The listing builds one solid part. Answer for the finished solid, in the listing's coordinates (mm). A direction names the side the tool comes from. Coordinates: 2 decimals unless noted, no trailing zeros. Order: outer loops, then holes, each group sorted by start corner. A loop starts at its lowest first (then second) coordinate and runs counter-clockwise, first axis right, second up. Notation, with made-up numbers: (56.5, 33.25) - (112.5, 33.25) arc R29 ccw to (112.5, 57.25) - close; hole circle Ø10 at (23.25, 70.5). An arc over 180 degrees is marked (long way). Use a Markdown table: item, result. Add a question column.
Item 1: The part is cut by section D-D, the plane z = -15. Give the vertices of the cut face in (x, y).
Item 2: The part is cut by section A-A, the plane x = 0. Give the vertices of the cut face in (y, z).
Item 3: The mould has two halves that part along X. Classify faces 1 (the flat face through (-1, 1, 51.235)), 2 (the flat face through (-17, 2, 18.867)), 3 (the cylindrical face through (31.29, 1.479, -44.397)), 4 (the flat face through (40, 2, 1)): released by +X, released by -X, zero draft, split by the parting line, or undercut.
Item 4: Flat-ended cylindrical pins translate along their axes: P1, Ø6, axis at x = 3, z = -2, coming from the -Y side; P2, Ø7, axis at x = 32.5, z = 42.5, coming from the +Y side; P3, Ø4, axis at x = -32.5, z = 42.5, coming from the -Y side. Find the tip coordinate at first contact, or state that the pin passes through.
Item 5: Find the intervals of material crossed by line 1 along X through (y, z) = (1.75, 42.5); line 2 along Z through (x, y) = (30, 1.75); line 3 along Y through (x, z) = (-5.5, 30.5), in increasing order.
Item 6: For faces 5 (the flat face through (0, 3, -39)), 6 (the flat face through (-1, 0, -12)), 7 (the flat face through (22.25, 2, -38)), determine the directions among +Z, -Z, +X, -X, +Y, -Y from which every point of the face is accessible in a straight line to the end or side of a thin tool.
Item 7: The part is cut by section B-B, the plane z = -39. Give the vertices of the cut face in (x, y).
Item 8: The part is cut by section C-C, the plane x = 16.5. Give the vertices of the cut face in (y, z), then the cut area to 3 significant figures.
from build123d import *

# Parameters (mm, degrees)
ESQUISSE1_R             = 65
DISQUE_DEPTH            = 3
ESQUISSE3_W             = 30.466369815
ESQUISSE3_H             = 200
COT_S_DEPTH             = 4
D_GAGEMENT_M3_52_D      = 3.9
D_GAGEMENT_M42_D        = 4.5
ESQUISSE15_W            = 89.863216067
ESQUISSE15_H            = 32.096215679
ENL_V_MAT_EXTRU_1_DEPTH = 34
D_GAGEMENT_M3_53_D      = 3.9
D_GAGEMENT_M3_53_DEPTH  = 3
D_GAGEMENT_M3_53_TIP    = 1.171678207
ESQUISSE22_W            = 113.248519978
ESQUISSE22_H            = 34.612898142
ESQUISSE22_W_2          = 51
ESQUISSE22_H_2          = 7
ESQUISSE22_W_3          = 65
ESQUISSE22_H_3          = 8
ENL_V_MAT_EXTRU_3_DEPTH = 10
ESQUISSE23_W            = 12
ESQUISSE23_H            = 14
ENL_V_MAT_EXTRU_4_DEPTH = 10
ESQUISSE24_W            = 18
ESQUISSE24_H            = 15
ENL_V_MAT_EXTRU_5_DEPTH = 10


with BuildPart() as part:
    # Esquisse1 → disque (new body)
    with BuildSketch(Plane(origin=(0, 0, 0), x_dir=(1, 0, 0), z_dir=(0, 1, 0))):
        Circle(ESQUISSE1_R)
    extrude(amount=DISQUE_DEPTH)

    # Esquisse3 → cotés (cut, through all)
    with BuildSketch(Plane(origin=(0, 3, 0), x_dir=(1, 0, 0), z_dir=(0, 1, 0))):
        with Locations((-55.233184908, 0)):
            Rectangle(ESQUISSE3_W, ESQUISSE3_H)
        with Locations((55.233184908, 0)):
            Rectangle(ESQUISSE3_W, ESQUISSE3_H)
    extrude(amount=-COT_S_DEPTH, mode=Mode.SUBTRACT)

    # Dégagement M3.52 (through all)
    with Locations(Plane(origin=(0, 3, 0), x_dir=(1, 0, 0), z_dir=(0, 1, 0))):
        with Locations((-30, -28.76524617)):
            d_gagement_m3_52 = Hole(D_GAGEMENT_M3_52_D / 2)

    # Symétrie1: Dégagement M3.52 across plane
    add(d_gagement_m3_52.mirror(Plane.ZY), mode=Mode.SUBTRACT)

    # Dégagement M42 (through all)
    with Locations(Plane(origin=(0, 3, 0), x_dir=(1, 0, 0), z_dir=(0, 1, 0))):
        with Locations((-32.5, 42.5), (32.5, 42.5), (32.5, -42.5), (-32.5, -42.5)):
            Hole(D_GAGEMENT_M42_D / 2)

    # Esquisse14 → Révolution1 (revolve)
    with BuildSketch(Plane.ZY):
        with BuildLine():
            Line((-35, 3), (-32, 3))
            Line((-32, 3), (-32, 26))
            ThreePointArc((-32, 26), (-34.050252532, 30.949747468), (-39, 33))
            Line((-39, 33), (-39, 30))
            ThreePointArc((-39, 30), (-36.171572875, 28.828427125), (-35, 26))
            Line((-35, 26), (-35, 3))
        make_face()
    revolve(axis=Axis((0, 3, -39), (0, 1, 0)))

    # Esquisse15 → Enlèv. mat.-Extru.1 (cut, through all)
    with BuildSketch(Plane.XZ):
        with Locations((-4.931608034, 67.282861669)):
            Rectangle(ESQUISSE15_W, ESQUISSE15_H)
    extrude(amount=-ENL_V_MAT_EXTRU_1_DEPTH, mode=Mode.SUBTRACT)

    # Dégagement M3.53
    with Locations(Plane(origin=(0, 0, 0), x_dir=(-1, 0, 0), z_dir=(0, -1, 0))):
        with Locations((-11.313708499, -8.367376915), (11.313708499, -36.367376915)):
            Hole(D_GAGEMENT_M3_53_D / 2, depth=D_GAGEMENT_M3_53_DEPTH)
            with Locations((0, 0, -(D_GAGEMENT_M3_53_DEPTH + D_GAGEMENT_M3_53_TIP / 2))):  # 118° drill point
                Cone(0, D_GAGEMENT_M3_53_D / 2, D_GAGEMENT_M3_53_TIP, mode=Mode.SUBTRACT)

    # Esquisse22 → Enlèv. mat.-Extru.3 (cut)
    with BuildSketch(Plane(origin=(0, 0, 0), x_dir=(-1, 0, 0), z_dir=(0, -1, 0))):
        with Locations((16.624259989, 68.541202901)):
            Rectangle(ESQUISSE22_W, ESQUISSE22_H)
        with Locations((0, -0.367376915)):
            Rectangle(ESQUISSE22_W_2, ESQUISSE22_H_2)
        with Locations((0, -44.367376915)):
            Rectangle(ESQUISSE22_W_2, ESQUISSE22_H_2)
        with Locations((0, 16.766315781)):
            Rectangle(ESQUISSE22_W_3, ESQUISSE22_H_3)
    extrude(amount=-ENL_V_MAT_EXTRU_3_DEPTH, mode=Mode.SUBTRACT)

    # Esquisse23 → Enlèv. mat.-Extru.4 (cut)
    with BuildSketch(Plane(origin=(0, 3, 0), x_dir=(1, 0, 0), z_dir=(0, 1, 0))):
        with Locations((-16.25, 38.367376915)):
            Rectangle(ESQUISSE23_W, ESQUISSE23_H)
        with Locations((16.25, 38.367376915)):
            Rectangle(ESQUISSE23_W, ESQUISSE23_H)
    extrude(amount=-ENL_V_MAT_EXTRU_4_DEPTH, mode=Mode.SUBTRACT)

    # Esquisse24 → Enlèv. mat.-Extru.5 (cut)
    with BuildSketch(Plane(origin=(0, 3, 0), x_dir=(1, 0, 0), z_dir=(0, 1, 0))):
        with Locations((-16.5, -11.367376915)):
            Rectangle(ESQUISSE24_W, ESQUISSE24_H)
        with Locations((16.5, -33.367376915)):
            Rectangle(ESQUISSE24_W, ESQUISSE24_H)
    extrude(amount=-ENL_V_MAT_EXTRU_5_DEPTH, mode=Mode.SUBTRACT)


solid = part.part
Solution:
| question | item | result |
|---|---|---|
| 1 | outline | (-40, 0) - (-32.5, 0) - (-32.5, 3) - (-40, 3) - close; (32.5, 0) - (40, 0) - (40, 3) - (32.5, 3) - close |
| 2 | outline | (0, -51.23) - (3, -51.23) - (3, -46) - (26, -46) arc R7 ccw to (26, -32) - (3, -32) - (3, -20.77) - (0, -20.77) - close; (0, -12.77) - (3, -12.77) - (3, -3.13) - (0, -3.13) - close; (0, 3.87) - (3, 3.87) - (3, 40.87) - (0, 40.87) - close; (0, 47.87) - (3, 47.87) - (3, 51.23) - (0, 51.23) - close; hole (3, -43) - (26, -43) arc R4 ccw to (26, -35) - (3, -35) - close |
| 3 | face 1 | zero draft |
| 3 | face 2 | undercut |
| 3 | face 3 | undercut |
| 3 | face 4 | released by +X |
| 4 | P1 | stops at y = 0 |
| 4 | P2 | stops at y = 3 |
| 4 | P3 | passes through |
| 5 | line 1 | x = -40 to -34.75, -30.25 to -25.5, 25.5 to 30.25, 34.75 to 40 |
| 5 | line 2 | z = -51.23 to -20.77, -12.77 to 26.82, 30.72 to 51.23 |
| 5 | line 3 | y = 0 to 3 |
| 6 | face 5 | none |
| 6 | face 6 | +Z, -Z, +X, -X, -Y |
| 6 | face 7 | +Y, -Y |
| 7 | outline | (-40, 0) - (-22.25, 0) - (-22.25, 3) - (-40, 3) - close; (-10.25, 0) - (10.25, 0) - (10.25, 3) - (7, 3) - (7, 26) arc R7 ccw to (-7, 26) - (-7, 3) - (-10.25, 3) - close; (22.25, 0) - (40, 0) - (40, 3) - (22.25, 3) - close; hole (-4, 3) - (4, 3) - (4, 26) arc R4 ccw to (-4, 26) - close |
| 8 | outline | (0, -51.23) - (3, -51.23) - (3, -45.37) - (0, -45.37) - close; (0, -31.37) - (3, -31.37) - (3, -20.77) - (0, -20.77) - close; (0, -12.77) - (3, -12.77) - (3, -3.13) - (0, -3.13) - close; (0, 3.87) - (3, 3.87) - (3, 25.87) - (0, 25.87) - close; (0, 47.87) - (3, 47.87) - (3, 51.23) - (0, 51.23) - close |
| 8 | area | 154 mm2 |
